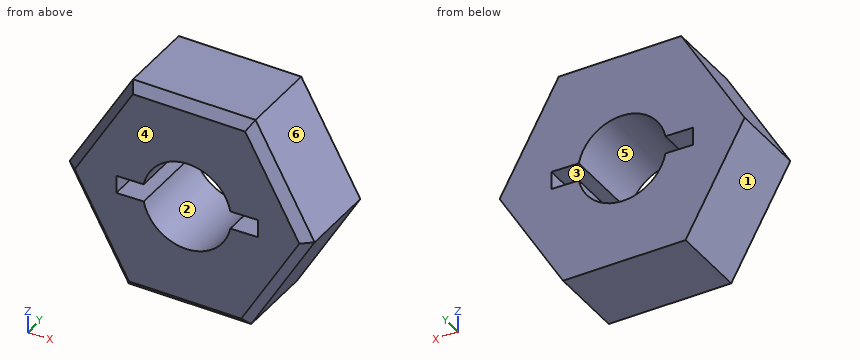
```python
from build123d import *

# Parameters (mm, degrees)
F0_DEPTH = 5
F1_R     = 2.5
F2_DEPTH = 36.487296
F6_SIZE  = 0.5
F3_W     = 8
F3_H     = 1
F4_DEPTH = 5.527664


with BuildPart() as f0:
    # F5 (on Front) → F0 (new body)
    with BuildSketch(Plane.XZ):
        Polygon((6.926796, -0.139655), (3.584342, 5.928954), (-3.342453, 6.068608), (-6.926796, 0.139655), (-3.584342, -5.928954), (3.342453, -6.068608), align=None)
    extrude(amount=F0_DEPTH)

    # F1 (on face) → F2 (cut)
    with BuildSketch(Plane.XZ):
        Circle(F1_R)
    extrude(amount=F2_DEPTH, mode=Mode.SUBTRACT)

    # F6
    f6_edges = [f0.edges().sort_by_distance(p)[0] for p in [
        (-5.255569, -5, -2.89465),
        (-5.134624, -5, 3.104131),
        (0.120944, -5, 5.998781),
        (5.255569, -5, 2.89465),
        (-0.120944, -5, -5.998781),
        (5.134624, -5, -3.104131),
    ]]
    chamfer(f6_edges, length=F6_SIZE)

    # F3 (on face) → F4 (cut)
    with BuildSketch(Plane.XZ):
        Rectangle(F3_W, F3_H)
    extrude(amount=F4_DEPTH, mode=Mode.SUBTRACT)


solid = f0.part
```
For this review, take the finished solid that the model builds, in its own axes (mm). Face numbers are marked on the shaded views. A direction names the side the tool comes from. Give positions to 0.01 mm unless a question says otherwise; leave off trailing zeros. Write each loop counter-clockwise with the first axis right and the second up, starting at its lowest first coordinate (ties: lowest second). Pieces come first, ordered by that corner, then holes. Notation, with made-up numbers: M 64.25,-35.5 L 119.25,-35.5 A29 cw 119.25,3.5 Z; hole C 76,-31 d10. An arc over 180 degrees is marked long. Answer as CSV lines item,"result".
1. For the marked faces 5 and 6, list the 3-axis set-ups (+Z, -Z, +X, -X, +Y, -Y) from which the entire face can be reached by the end or side of a thin tool; tool diameter is ignored.
Findings:
face 5,"+Y, -Y"
face 6,"+Z, +X, +Y, -Y"
2. Consider section B-B, the plane z = 1.5. Write out the cut boundary in (x, y), then the cut area to 3 significant figures.
Findings:
outline,"M -6.1,-4.5 L -5.52,-5 L -2,-5 L -2,0 L -6.1,0 Z; M 2,-5 L 5.45,-5 L 6.02,-4.5 L 6.02,0 L 2,0 Z"
area,"40.4 mm2"
3. Consider section C-C, the plane x = -1. Write out the cut boundary in (y, z).
Findings:
outline,"M -5,-5.48 L -4.5,-5.98 L 0,-5.98 L 0,-2.29 L -5,-2.29 Z; M -5,2.29 L 0,2.29 L 0,6.02 L -4.5,6.02 L -5,5.52 Z"
4. Draft analysis for pull direction X (two halves, no side actions). For the marked faces 1, 2, 3 and 4, state which applies: +X half, -X half, draft (parallel to the pull), parting line (faces both ways), or undercut.
Findings:
face 1,"-X half"
face 2,"undercut"
face 3,"undercut"
face 4,"draft"
5. Consider section D-D, the plane x = -5.25. Write out the cut boundary in (y, z), then the cut area to 3 significant figures.
Findings:
outline,"M -5,-1.87 L -4.5,-2.9 L 0,-2.9 L 0,2.91 L -4.5,2.91 L -5,1.95 Z"
area,"28.6 mm2"
6. Wall thickness on line 1 (X direction, y = -1.4, z = -1); line 2 (Z direction, x = 2.25, y = -1.2); line 3 (X direction, y = -0.8, z = -2): over which ranges is each line inside the solid? List them lowest first.
Findings:
line 1,"x = -6.3 to -2.29, 2.29 to 6.41"
line 2,"z = -6.05 to -1.09, 1.09 to 5.96"
line 3,"x = -5.75 to -1.5, 1.5 to 5.8"
7. For pin 1 (2 mm diameter, centred on y = -3, z = 2.5, fed in from +X); pin 2 (3 mm diameter, centred on y = -1, z = -4, fed in from +X); pin 3 (3 mm diameter, centred on y = -1, z = 1.5, fed in from +X), all flat-tipped, find the tip position at first contact; note any pin that passes through.
Findings:
pin 1,"stops at x = 6.02"
pin 2,"stops at x = 5.5"
pin 3,"stops at x = 6.85"
8. Consider section A-A, the plane y = -0.4. Write out the cut boundary in (x, z).
Findings:
outline,"M -6.93,0.14 L -3.58,-5.93 L 3.34,-6.07 L 6.93,-0.14 L 3.58,5.93 L -3.34,6.07 Z; hole M -4,-0.5 L -2.45,-0.5 A2.5 ccw 2.45,-0.5 L 4,-0.5 L 4,0.5 L 2.45,0.5 A2.5 ccw -2.45,0.5 L -4,0.5 Z"
